Check sheet for the modelled part. Datum: model origin and axes. Units: mm. Give positions to 0.01 mm unless a question says otherwise; leave off trailing zeros. Write each loop counter-clockwise with the first axis right and the second up, starting at its lowest first coordinate (ties: lowest second). Pieces come first, ordered by that corner, then holes.
from build123d import *

# Parameters (mm, degrees)
F0_R     = 11.1125
F1_DEPTH = 25.4


with BuildPart() as f1:
    # F0 (on Right) → F1 (new body)
    with BuildSketch(Plane.YZ):
        with BuildLine():
            Line((76.2, 38.1), (-38.1, 38.1))
            Line((-38.1, 38.1), (-69.85, 12.7))
            ThreePointArc((-69.85, 12.7), (-76.2, 0), (-69.85, -12.7))
            Line((-69.85, -12.7), (-38.1, -38.1))
            Line((-38.1, -38.1), (76.2, -38.1))
            Line((76.2, -38.1), (76.2, 38.1))
        make_face()
        with Locations((-55.88, 0)):
            Circle(F0_R, mode=Mode.SUBTRACT)
    extrude(amount=F1_DEPTH)


solid = f1.part
1) Draft check along Z on faces 1 (the cylindrical face through (12.5, -76.2, 0.2)), 2 (the flat face through (25.4, 16, 1)), 3 (the flat face through (12.52, -54.2, -25.22)), 4 (the cylindrical face through (12.52, -45.28, 3.34)). Enter one of: +Z half, -Z half, draft (parallel to the pull), parting line (faces both ways), or undercut.
2) Scan lines: L1, parallel to Z at x = 13.5, y = -56; L2, parallel to Z at x = 8.5, y = -66; L3, parallel to Y at x = 15.25, z = -6. Record each from-to range of solid material in increasing order.
3) Sectioned sample at D-D on z = 23. Record the boundary of the cut face in (x, y) (3 decimals), then the cut area to 3 significant figures.
4) Sectioned sample at A-A on z = 0. Record the boundary of the cut face in (x, y).
5) Sectioned sample at B-B on y = -51.5. Record the boundary of the cut face in (x, z), then the cut area to 3 significant figures.
6) Gauge pin test, flat ends, axial feed: pin 1 (5 mm diameter, centred on x = 19, z = -4, fed in from -Y); pin 2 (1.5 mm diameter, centred on x = 5.5, z = 21, fed in from -Y); pin 3 (18 mm diameter, centred on y = -55.88, z = 0, fed in from +X). Record the tip position at first contact, or that the pin passes through.
Answers below:
1. face 1: parting line
1. face 2: draft
1. face 3: -Z half
1. face 4: undercut
2. L1: z = -23.78 to -11.11, 11.11 to 23.78
2. L2: z = -15.78 to -4.59, 4.59 to 15.78
2. L3: y = -75.02 to -65.23, -46.53 to 76.2
3. outline: (0, -56.975) - (25.4, -56.975) - (25.4, 76.2) - (0, 76.2) - close
3. area: 3,380 mm2
4. outline: (0, -76.2) - (25.4, -76.2) - (25.4, -66.99) - (0, -66.99) - close; (0, -44.77) - (25.4, -44.77) - (25.4, 76.2) - (0, 76.2) - close
5. outline: (0, -27.38) - (25.4, -27.38) - (25.4, -10.21) - (0, -10.21) - close; (0, 10.21) - (25.4, 10.21) - (25.4, 27.38) - (0, 27.38) - close
5. area: 872 mm2
6. pin 1: stops at y = -76.13
6. pin 2: stops at y = -60.41
6. pin 3: passes through
